```python
from build123d import *

# Parameters (mm, degrees)
F1_DEPTH = 5
F6_DEPTH = 1
F8_DEPTH = 3
F9_DEPTH = 3


with BuildPart() as f1:
    # F0 (on Top) → F1 (new body)
    with BuildSketch(Plane.XY):
        Polygon((15, 0), (-15, 0), (0, -26), align=None)
    extrude(amount=F1_DEPTH)

    # F1_face (on face) → F4 section 0
    with BuildSketch(Plane(origin=(0, -8.6666666667, 5), x_dir=(1, 0, 0), z_dir=(0, 0, 1))):
        Polygon((15, 8.6666666667), (-15, 8.6666666667), (0, -17.3333333333), align=None)
    # F3 (on offset) → F4 section 1
    with BuildSketch(Plane.XY.offset(7)):
        Polygon((0, -21.9977783947), (11.5371798431, -2), (-11.5371798431, -2), align=None)
    loft()

    # F6 (cut): a face of the model
    f6_faces = [f1.faces().sort_by_distance(p)[0] for p in [
        (0, -8.6659261316, 7),
    ]]
    extrude(f6_faces, amount=-F6_DEPTH, mode=Mode.SUBTRACT)

    # F7 (on face) → F8 (cut)
    with BuildSketch(Plane.XY.offset(6)):
        Polygon((0, -21.3974451539), (11.0177568196, -2.3), (-11.0177568196, -2.3), align=None)
    extrude(amount=-F8_DEPTH, mode=Mode.SUBTRACT)

    # F5 (on face) → F9 (cut, through all)
    with BuildSketch(Plane(origin=(0, 0, 0), x_dir=(1, 0, 0), z_dir=(0, 0, -1))):
        Polygon((0, 22.3980005552), (-11.8834618588, 1.8), (11.8834618588, 1.8), align=None)
    extrude(amount=-F9_DEPTH, mode=Mode.SUBTRACT)


solid = f1.part
```
The listing builds one solid part. Answer for the finished solid, in the listing's coordinates (mm). A direction names the side the tool comes from. Give positions to 0.01 mm unless a question says otherwise; leave off trailing zeros. Write each loop counter-clockwise with the first axis right and the second up, starting at its lowest first coordinate (ties: lowest second). Pieces come first, ordered by that corner, then holes. Notation, with made-up numbers: (78, -36.5) -> (135, -36.5) arc R14 ccw to (135, -19.5) -> close; hole circle Ø10 at (40.25, 0). An arc over 180 degrees is marked (long way). Use one line per item in the form item = value.
1) Straight lines are drawn through the part: probe 1 along Y at (x, z) = (5, 3.5); probe 2 along X at (y, z) = (-6, 0.75); probe 3 along Y at (x, z) = (-10, 5.75). For each, find the intervals that lie inside material, in ascending order.
Result:
probe_1 = -17.33 to -12.73, -2.3 to 0
probe_2 = -11.54 to -9.46, 9.46 to 11.54
probe_3 = -7.17 to -4.06, -2.3 to -0.75
2) Section B-B on z = 2 is taken. Write down the section's boundary in (x, y), plus the area to 3 significant figures.
Result:
outline = (-15, 0) -> (0, -26) -> (15, 0) -> close; hole (-11.88, -1.8) -> (0, -22.4) -> (11.88, -1.8) -> close
area = 145 mm²
3) A tool of negligible diameter and unlimited length cuts with its end or side. For faces 1 (the flat face through (-6, -12, 1)), 2 (the flat face through (-5.85, -11.86, 6.51)), 3 (the flat face through (5.432, -11.982, 4.521)), from which of +Z, -Z, +X, -X, +Y, -Y can it reach the whole face along a straight path? Write none if from no direction.
Result:
face_1 = -Z
face_2 = +Z
face_3 = +Z, -Z
4) For a pull along Y with two mould halves and no side action, classify faces 4 (the flat face through (-5.586, -11.715, 4.521)), 5 (the flat face through (0, 0, 2)), 6 (the flat face through (-7, -11, 0)), 7 (the flat face through (-1, -2, 3)) as +Y half, -Y half, draft (parallel to the pull), parting line (faces both ways), or undercut.
Result:
face_4 = undercut
face_5 = +Y half
face_6 = draft
face_7 = undercut
5) Section A-A on z = 3.75 is taken. Write down the section's boundary in (x, y), plus the area to 3 significant figures.
Result:
outline = (-15, 0) -> (0, -26) -> (15, 0) -> close; hole (-11.02, -2.3) -> (0, -21.4) -> (11.02, -2.3) -> close
area = 180 mm²
6) This flat-tipped pin is pushed along its axis until it touches: P1, Ø1.5, axis at x = -0.5, z = 4, coming from the -Y side. Where does it stop, or does it pass through?
Result:
P1 = -26
